Source: three-view drawing plus pictorial views. Frame: mm from the lowest corner of the part. Give positions to 0.01 mm unless a question says otherwise; leave off trailing zeros. Loops run counter-clockwise (first coordinate to the right, second up) from the corner with the lowest first, then second, coordinate; pieces in that order, holes last. Notation, with made-up numbers: M -4.5,69.5 L 43.5,69.5 A13 ccw 43.5,78.5 Z; hole C 66.5,85 d3. An arc over 180 degrees is marked long. Write item = value, one per line.
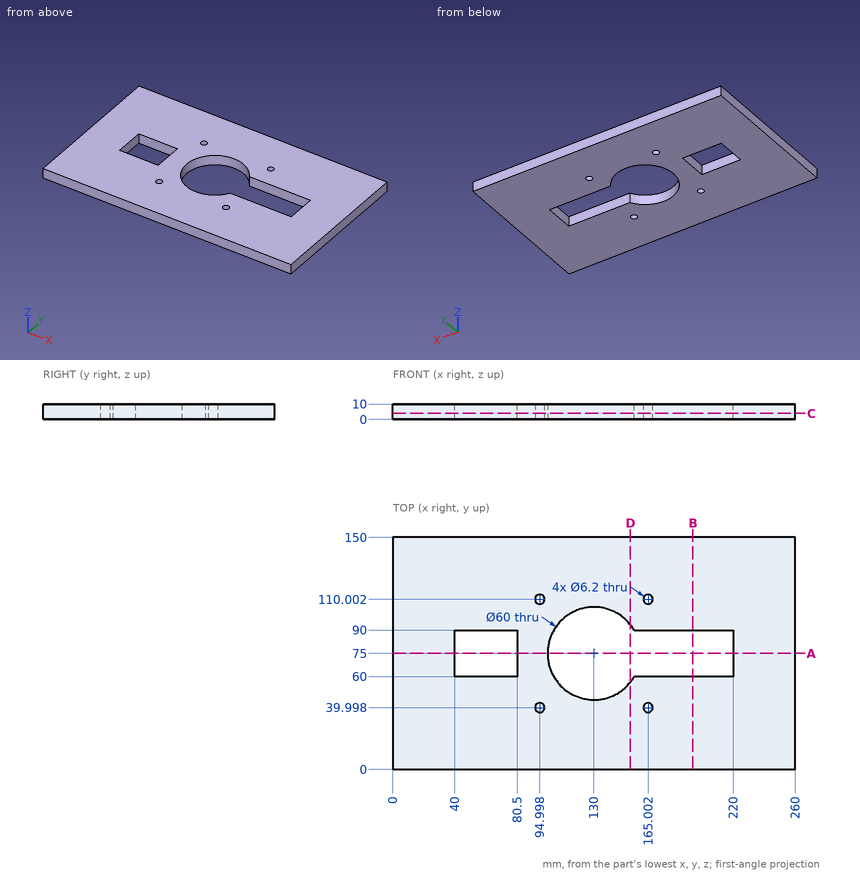
1. Cut plane B-B, the plane x = 194. Return the cut outline in (y, z), then the cut area to 3 significant figures.
Derived:
outline = M 0,0 L 60,0 L 60,10 L 0,10 Z; M 90,0 L 150,0 L 150,10 L 90,10 Z
area = 1,200 mm²
2. First-contact query: pin 1 Ø12 at (x, y) = (120, 123) entering from -Z; pin 2 Ø3.5 at (x, y) = (165, 40) entering from +Z. Flat tips, straight axial feed; report the tip coordinate or a pass-through.
Derived:
pin_1 = 0
pin_2 = through
3. Material intervals for probe 1 along Y at (x, z) = (202.5, 4); probe 2 along X at (y, z) = (42, 8.5) (1 decimal); probe 3 along X at (y, z) = (75, 2.5), sorted ascending. Write a range as from..to.
Derived:
probe_1 = 0..60, 90..150
probe_2 = 0..92.6, 97.4..162.6, 167.4..260
probe_3 = 0..40, 80.5..100, 220..260
4. Cut plane C-C, the plane z = 4. Return the cut outline in (x, y).
Derived:
outline = M 0,0 L 260,0 L 260,150 L 0,150 Z; hole M 40,60 L 80.5,60 L 80.5,90 L 40,90 Z; hole C 95,40 d6.2; hole C 95,110 d6.2; hole M 155.98,60 L 220,60 L 220,90 L 155.98,90 A30 ccw long Z; hole C 165,40 d6.2; hole C 165,110 d6.2
5. Cut plane D-D, the plane x = 153.5. Return the cut outline in (y, z).
Derived:
outline = M 0,0 L 56.35,0 L 56.35,10 L 0,10 Z; M 93.65,0 L 150,0 L 150,10 L 93.65,10 Z
6. Cut plane A-A, the plane y = 75. Return the cut outline in (x, z).
Derived:
outline = M 0,0 L 40,0 L 40,10 L 0,10 Z; M 80.5,0 L 100,0 L 100,10 L 80.5,10 Z; M 220,0 L 260,0 L 260,10 L 220,10 Z
